from build123d import *

# Parameters (mm, degrees)
SKETCH1_W           = 8.153779141
SKETCH1_H           = 12.8
SKETCH1_H_2         = 24.7
SKETCH1_W_2         = 40
SKETCH1_W_3         = 7.846220859
BOSS_EXTRUDE1_DEPTH = 20
SKETCH4_W           = 20
SKETCH4_H           = 24.7
CUT_EXTRUDE1_DEPTH  = 8
SKETCH5_W           = 20
SKETCH5_H           = 24.7
CUT_EXTRUDE2_DEPTH  = 8
SKETCH6_W           = 20
SKETCH6_H           = 10.1
CUT_EXTRUDE3_DEPTH  = 8
SKETCH7_W           = 20
SKETCH7_H           = 10.1
CUT_EXTRUDE4_DEPTH  = 8


with BuildPart() as part:
    # Sketch1 → Boss-Extrude1 (new body)
    with BuildSketch(Plane.XY):
        with Locations((4.076889571, 31.1)):
            Rectangle(SKETCH1_W, SKETCH1_H)
        with Locations((4.076889571, 12.35)):
            Rectangle(SKETCH1_W, SKETCH1_H_2)
        with Locations((28.153779141, 31.1)):
            Rectangle(SKETCH1_W_2, SKETCH1_H)
        with Locations((28.153779141, 12.35)):
            Rectangle(SKETCH1_W_2, SKETCH1_H_2)
        with Locations((52.076889571, 31.1)):
            Rectangle(SKETCH1_W_3, SKETCH1_H)
        with Locations((52.076889571, 12.35)):
            Rectangle(SKETCH1_W_3, SKETCH1_H_2)
    extrude(amount=BOSS_EXTRUDE1_DEPTH)

    # Sketch4 → Cut-Extrude1 (cut)
    with BuildSketch(Plane.ZY):
        with Locations((10, 12.35)):
            Rectangle(SKETCH4_W, SKETCH4_H)
    extrude(amount=-CUT_EXTRUDE1_DEPTH, mode=Mode.SUBTRACT)

    # Sketch5 → Cut-Extrude2 (cut)
    with BuildSketch(Plane(origin=(56, 0, 0), x_dir=(0, 0, -1), z_dir=(1, 0, 0))):
        with Locations((-10, 12.35)):
            Rectangle(SKETCH5_W, SKETCH5_H)
    extrude(amount=-CUT_EXTRUDE2_DEPTH, mode=Mode.SUBTRACT)

    # Sketch6 → Cut-Extrude3 (cut)
    with BuildSketch(Plane(origin=(56, 0, 0), x_dir=(0, 0, -1), z_dir=(1, 0, 0))):
        with Locations((-10, 32.45)):
            Rectangle(SKETCH6_W, SKETCH6_H)
    extrude(amount=-CUT_EXTRUDE3_DEPTH, mode=Mode.SUBTRACT)

    # Sketch7 → Cut-Extrude4 (cut)
    with BuildSketch(Plane.ZY):
        with Locations((10, 32.45)):
            Rectangle(SKETCH7_W, SKETCH7_H)
    extrude(amount=-CUT_EXTRUDE4_DEPTH, mode=Mode.SUBTRACT)


solid = part.part
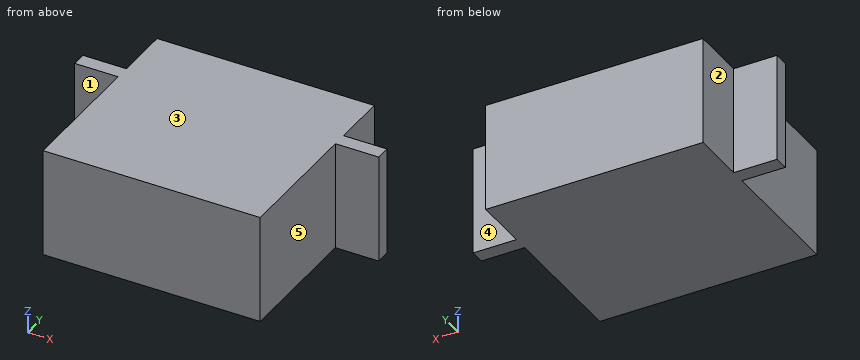
The model under review builds one solid part; all positions refer to its coordinate system, in mm. Face numbers are marked on the shaded views. A direction names the side the tool comes from. Round coordinates to 2 decimals unless told otherwise and drop trailing zeros. Write each loop counter-clockwise with the first axis right and the second up, starting at its lowest first coordinate (ties: lowest second). Pieces come first, ordered by that corner, then holes. Notation, with made-up numbers: M -28.75,48.5 L -15.75,48.5 A17 cw -15.75,73.5 Z; hole C -17,89.25 d1. An arc over 180 degrees is marked long. Answer as CSV lines item,"result". Start each with the question number.
Q1. Clearance check with flat-ended pins moving along their axes: P1, Ø1.5, axis at y = 14.5, z = 14.5, coming from the -X side; P2, Ø6, axis at y = 9, z = 8.5, coming from the +X side; P3, Ø4, axis at x = 50.5, z = 11, coming from the +Y side. State where each tip first meets the part, or that it passes through.
Q2. Wall thickness on line 1 along X through (y, z) = (28, 10.25); line 2 along Y through (x, z) = (49.5, 18.5): over which ranges is each line inside the solid? List them lowest first.
Q3. Tool access review of the marked faces 1, 2, 3, 4 and 5: name each direction out of +Z, -Z, +X, -X, +Y, -Y from which nothing blocks a thin tool from reaching the whole face with its end or side.
Q4. Consider section C-C, the plane y = 21.5. Give the boundary of the cut face in (x, z).
Q5. Consider section B-B, the plane x = 52.5. Give the boundary of the cut face in (y, z).
Q6. Consider section A-A, the plane z = 16. Give the boundary of the cut face in (x, y), then the cut area to 3 significant figures.
Result set:
1,P1,"stops at x = 8"
1,P2,"stops at x = 48"
1,P3,"stops at y = 27.4"
2,line 1,"x = 8 to 48"
2,line 2,"y = 24.7 to 27.4"
3,face 1,"+Z, -Z, -X, -Y"
3,face 2,"+Z, -Z, -X, +Y"
3,face 3,"+Z, +X, -X, +Y, -Y"
3,face 4,"+Z, -Z, +X, +Y"
3,face 5,"+Z, -Z, +X, -Y"
4,outline,"M 8,0 L 48,0 L 48,20 L 8,20 Z"
5,outline,"M 24.7,0 L 27.4,0 L 27.4,20 L 24.7,20 Z"
6,outline,"M 0,24.7 L 8,24.7 L 8,0 L 48,0 L 48,24.7 L 56,24.7 L 56,27.4 L 48,27.4 L 48,37.5 L 8,37.5 L 8,27.4 L 0,27.4 Z"
6,area,"1,540 mm²"
